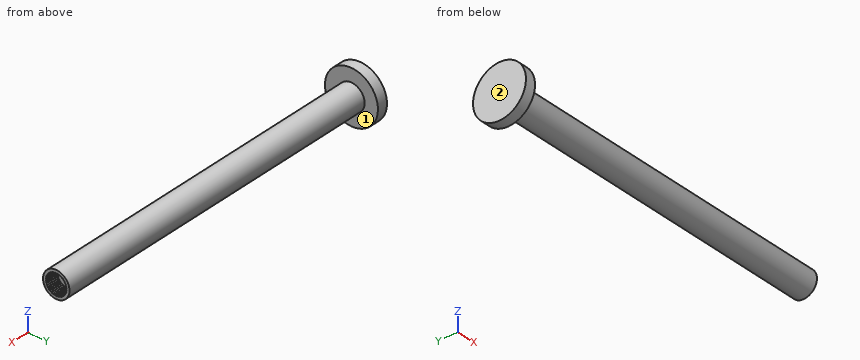
```python
from build123d import *

# Parameters (mm, degrees)
SKETCH1_R           = 6.35
BOSS_EXTRUDE1_DEPTH = 2.54
SKETCH2_R           = 3.175
BOSS_EXTRUDE2_DEPTH = 82.55
SKETCH3_R           = 2.3495
CUT_EXTRUDE1_DEPTH  = 3.175
SKETCH4_R           = 0.1524
CUT_EXTRUDE2_DEPTH  = 3.175


with BuildPart() as part:
    # Sketch1 → Boss-Extrude1 (new body)
    with BuildSketch(Plane(origin=(0, 0, 0), x_dir=(0, 0, -1), z_dir=(1, 0, 0))):
        Circle(SKETCH1_R)
    extrude(amount=BOSS_EXTRUDE1_DEPTH)

    # Sketch2 → Boss-Extrude2 (add)
    with BuildSketch(Plane(origin=(2.54, 0, 0), x_dir=(0, 0, -1), z_dir=(1, 0, 0))):
        Circle(SKETCH2_R)
    extrude(amount=BOSS_EXTRUDE2_DEPTH)

    # Sketch3 → Cut-Extrude1 (cut)
    with BuildSketch(Plane(origin=(85.09, 0, 0), x_dir=(0, 0, -1), z_dir=(1, 0, 0))):
        Circle(SKETCH3_R)
    extrude(amount=-CUT_EXTRUDE1_DEPTH, mode=Mode.SUBTRACT)

    # Sketch4 → Cut-Extrude2 (cut)
    with BuildSketch(Plane(origin=(85.09, 0, 0), x_dir=(0, 0, -1), z_dir=(1, 0, 0))):
        with Locations((1.261294478, 1.982242793)):
            Circle(SKETCH4_R)
        with Locations((1.555856941, 1.760528167)):
            Circle(SKETCH4_R)
        with Locations((1.812109043, 1.495463496)):
            Circle(SKETCH4_R)
        with Locations((2.023741005, 1.19357555)):
            Circle(SKETCH4_R)
        with Locations((2.185541748, 0.862297813)):
            Circle(SKETCH4_R)
        with Locations((2.293527199, 0.509787442)):
            Circle(SKETCH4_R)
        with Locations((2.345038399, 0.144724412)):
            Circle(SKETCH4_R)
        with Locations((2.338806971, -0.223902213)):
            Circle(SKETCH4_R)
        with Locations((2.274986353, -0.587015623)):
            Circle(SKETCH4_R)
        with Locations((2.155148021, -0.93567476)):
            Circle(SKETCH4_R)
        with Locations((1.982242793, -1.261294478)):
            Circle(SKETCH4_R)
        with Locations((1.760528167, -1.555856941)):
            Circle(SKETCH4_R)
        with Locations((1.495463496, -1.812109043)):
            Circle(SKETCH4_R)
        with Locations((1.19357555, -2.023741005)):
            Circle(SKETCH4_R)
        with Locations((0.862297813, -2.185541748)):
            Circle(SKETCH4_R)
        with Locations((0.509787442, -2.293527199)):
            Circle(SKETCH4_R)
        with Locations((0.144724412, -2.345038399)):
            Circle(SKETCH4_R)
        with Locations((-0.223902213, -2.338806971)):
            Circle(SKETCH4_R)
        with Locations((-0.587015623, -2.274986353)):
            Circle(SKETCH4_R)
        with Locations((-0.93567476, -2.155148021)):
            Circle(SKETCH4_R)
        with Locations((-1.261294478, -1.982242793)):
            Circle(SKETCH4_R)
        with Locations((-1.555856941, -1.760528167)):
            Circle(SKETCH4_R)
        with Locations((-1.812109043, -1.495463496)):
            Circle(SKETCH4_R)
        with Locations((-2.023741005, -1.19357555)):
            Circle(SKETCH4_R)
        with Locations((-2.185541748, -0.862297813)):
            Circle(SKETCH4_R)
        with Locations((-2.293527199, -0.509787442)):
            Circle(SKETCH4_R)
        with Locations((-2.345038399, -0.144724412)):
            Circle(SKETCH4_R)
        with Locations((-2.338806971, 0.223902213)):
            Circle(SKETCH4_R)
        with Locations((-2.274986353, 0.587015623)):
            Circle(SKETCH4_R)
        with Locations((-2.155148021, 0.93567476)):
            Circle(SKETCH4_R)
        with Locations((-1.982242793, 1.261294478)):
            Circle(SKETCH4_R)
        with Locations((-1.760528167, 1.555856941)):
            Circle(SKETCH4_R)
        with Locations((-1.495463496, 1.812109043)):
            Circle(SKETCH4_R)
        with Locations((-1.19357555, 2.023741005)):
            Circle(SKETCH4_R)
        with Locations((-0.862297813, 2.185541748)):
            Circle(SKETCH4_R)
        with Locations((-0.509787442, 2.293527199)):
            Circle(SKETCH4_R)
        with Locations((-0.144724412, 2.345038399)):
            Circle(SKETCH4_R)
        with Locations((0.223902213, 2.338806971)):
            Circle(SKETCH4_R)
        with Locations((0.587015623, 2.274986353)):
            Circle(SKETCH4_R)
        with Locations((0.93567476, 2.155148021)):
            Circle(SKETCH4_R)
    extrude(amount=-CUT_EXTRUDE2_DEPTH, mode=Mode.SUBTRACT)


solid = part.part
```
Input: part model. Units: mm. Frame: model coordinates. Face numbers are marked on the shaded views. A direction names the side the tool comes from. Give positions to 0.01 mm unless a question says otherwise; leave off trailing zeros. Write each loop counter-clockwise with the first axis right and the second up, starting at its lowest first coordinate (ties: lowest second). Pieces come first, ordered by that corner, then holes. Notation, with made-up numbers: (-34.75, -38) - (24.25, -38) arc R36 ccw to (24.25, -3) - close; hole circle Ø11 at (18.25, 8). An arc over 180 degrees is marked (long way). Write item = value, one per line. Start each with the question number.
1. First-contact query: pin 1 Ø2 at (x, z) = (53, -1) entering from -Y (3 decimals); pin 2 Ø5 at (x, z) = (66, 3.5) entering from -Y; pin 3 Ø6 at (x, y) = (51.5, 2) entering from -Z (3 decimals). Flat tips, straight axial feed; report the tip coordinate or a pass-through.
2. Section query B-B, the plane z = 5.5. Output: boundary loops of the cut face in (x, y), then the cut area to 3 significant figures.
3. Access query for the marked faces 1 and 2. Directions: +Z, -Z, +X, -X, +Y, -Y. A direction counts if a zero-diameter tool reaches every point of the face in a straight line with its end or side. Return the directions, or none.
4. Ray query, L1, parallel to X at y = 4, z = 3.5; L2, parallel to Z at x = 25.5, y = 2.5; L3, parallel to Z at x = 8.5, y = -2.25. Return the intervals inside material, ascending.
5. Section query A-A, the plane x = 77. Output: boundary loops of the cut face in (y, z) (3 decimals).
Check sheet entries:
q1.pin_1 = -3.175
q1.pin_2 = -3.01
q1.pin_3 = -3.175
q2.outline = (0, -3.17) - (2.54, -3.17) - (2.54, 3.17) - (0, 3.17) - close
q2.area = 16.1 mm2
q3.face_1 = +X
q3.face_2 = +Z, -Z, -X, +Y, -Y
q4.L1 = 0 to 2.54
q4.L2 = -1.96 to 1.96
q4.L3 = -2.24 to 2.24
q5.outline = circle Ø6.35 at (0, 0)
